Geometry: final body of the model. Coordinates: model frame, mm. Coordinates: 2 decimals unless noted, no trailing zeros. Order: outer loops, then holes, each group sorted by start corner. A loop starts at its lowest first (then second) coordinate and runs counter-clockwise, first axis right, second up. Notation, with made-up numbers: M 26.25,51.5 L 75.25,51.5 A24 ccw 75.25,83.5 Z; hole C 28,64.5 d2. An arc over 180 degrees is marked long. Use CSV: the item, a comma, the result in double quotes. Start each with the question number.
Q1. First-contact query: P1, Ø2, axis at x = 30.5, z = -17.5, coming from the +Y side. Flat tip, straight axial feed; report the tip coordinate or a pass-through.
Q2. Section query A-A, the plane x = 12.7. Output: boundary loops of the cut face in (y, z).
Q3. Mould query, pull axis Z, two halves, no side actions, for faces 1 (the face through (-1, -6, 30.48)), 2 (the face through (-1, -12.7, 0)), 3 (the face through (-31.696, -6.261, -23.836)), 4 (the face through (7.663, -6.439, 0.222)). Classes: +Z half, -Z half, draft (parallel to the pull), parting line (faces both ways), or undercut.
Q4. Section query D-D, the plane y = -8. Output: boundary loops of the cut face in (x, z) (1 decimal).
Q5. Ray query, probe 1 along Z at (x, y) = (-28.5, -2.5); probe 2 along Z at (x, y) = (-25.5, -8); probe 3 along Z at (x, y) = (12.7, -7). Return the intervals inside material, ascending.
Q6. Section query B-B, the plane z = 0. Output: boundary loops of the cut face in (x, y) (3 decimals).
Q7. Section query C-C, the plane x = -30. Output: boundary loops of the cut face in (y, z), and give its area (3 significant figures).
from build123d import *

# Parameters (mm, degrees)
F0_W     = 82.55
F0_H     = 60.96
F1_DEPTH = 12.7
F3_D     = 10.0838
F5_D     = 6.7564


with BuildPart() as f1:
    # F0 (on Front) → F1 (new body)
    with BuildSketch(Plane.XZ):
        Rectangle(F0_W, F0_H)
    extrude(amount=F1_DEPTH)

    # F3 (through all)
    with Locations(Plane(origin=(0, 0, 0), x_dir=(-1, 0, 0), z_dir=(0, 1, 0))):
        with Locations((-12.7, 0)):
            Hole(F3_D / 2)

    # F5 (through all)
    with Locations(Plane.XZ.offset(12.7)):
        with Locations((-28.575, 22.5425), (-28.575, -22.5425)):
            Hole(F5_D / 2)


solid = f1.part
Responses:
1,P1,"stops at y = 0"
2,outline,"M -12.7,-30.48 L 0,-30.48 L 0,-5.04 L -12.7,-5.04 Z; M -12.7,5.04 L 0,5.04 L 0,30.48 L -12.7,30.48 Z"
3,face 1,"+Z half"
3,face 2,"draft"
3,face 3,"undercut"
3,face 4,"undercut"
4,outline,"M -41.3,-30.5 L 41.3,-30.5 L 41.3,30.5 L -41.3,30.5 Z; hole C -28.6,-22.5 d6.8; hole C -28.6,22.5 d6.8; hole C 12.7,0 d10.1"
5,probe 1,"z = -30.48 to -25.92, -19.17 to 19.17, 25.92 to 30.48"
5,probe 2,"z = -30.48 to -23.94, -21.14 to 21.14, 23.94 to 30.48"
5,probe 3,"z = -30.48 to -5.04, 5.04 to 30.48"
6,outline,"M -41.275,-12.7 L 7.658,-12.7 L 7.658,0 L -41.275,0 Z; M 17.742,-12.7 L 41.275,-12.7 L 41.275,0 L 17.742,0 Z"
7,outline,"M -12.7,-30.48 L 0,-30.48 L 0,-25.61 L -12.7,-25.61 Z; M -12.7,-19.48 L 0,-19.48 L 0,19.48 L -12.7,19.48 Z; M -12.7,25.61 L 0,25.61 L 0,30.48 L -12.7,30.48 Z"
7,area,"619 mm²"
